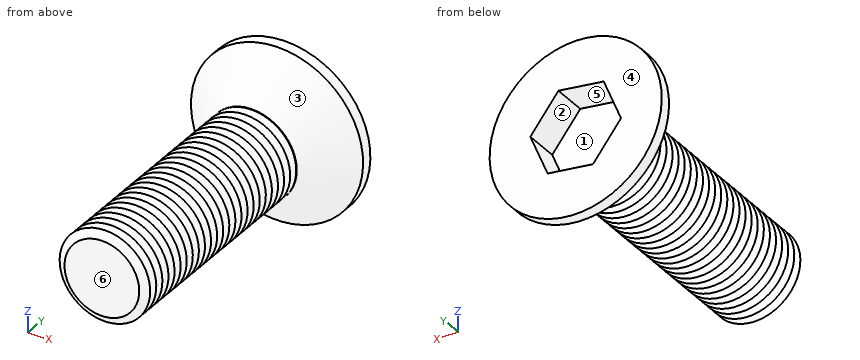
```python
from build123d import *

# Parameters (mm, degrees)
CUT_EXTRUDE_1_DEPTH = 3


with BuildPart() as part:
    # 草图1 → 旋转1 (revolve)
    with BuildSketch(Plane.XY, mode=Mode.PRIVATE) as revolve_1_sk:
        Polygon((7.6, 25), (0, 25), (0, 0), (3.3, 0), (4, 0.416910771), (3.3, 0.833821542), (4, 1.250732313), (3.3, 1.667643084), (4, 2.084553856), (3.3, 2.501464627), (4, 2.918375398), (3.3, 3.335286169), (4, 3.75219694), (3.3, 4.169107711), (4, 4.586018482), (3.3, 5.002929253), (4, 5.419840024), (3.3, 5.836750796), (4, 6.253661567), (3.3, 6.670572338), (4, 7.087483109), (3.3, 7.50439388), (4, 7.921304651), (3.3, 8.338215422), (4, 8.755126193), (3.3, 9.172036964), (4, 9.588947736), (3.3, 10.005858507), (4, 10.422769278), (3.3, 10.839680049), (4, 11.25659082), (3.3, 11.673501591), (4, 12.090412362), (3.3, 12.507323133), (4, 12.924233904), (3.3, 13.341144675), (4, 13.758055447), (3.3, 14.174966218), (4, 14.591876989), (3.3, 15.00878776), (4, 15.425698531), (3.3, 15.842609302), (4, 16.259520073), (3.3, 16.676430844), (4, 17.093341615), (3.3, 17.510252387), (4, 17.927163158), (3.3, 18.344073929), (4, 18.7609847), (3.3, 19.177895471), (4, 19.594806242), (3.3, 20.011717013), (4, 20.428627784), (4, 20.5), (7.6, 24), align=None)
    revolve(revolve_1_sk.sketch.rotate(Axis((0, 20.5, 0), (0, 1, 0)), 270), axis=Axis((0, 20.5, 0), (0, 1, 0)))

    # 草图3 → 切除-拉伸1 (cut)
    with BuildSketch(Plane(origin=(0, 25, 0), x_dir=(1, 0, 0), z_dir=(0, 1, 0))):
        Polygon((4.003980009, -0.549069595), (2.477498223, 3.193013606), (-1.526481787, 3.742083202), (-4.003980009, 0.549069595), (-2.477498223, -3.193013606), (1.526481787, -3.742083202), align=None)
    extrude(amount=-CUT_EXTRUDE_1_DEPTH, mode=Mode.SUBTRACT)


solid = part.part
```
Check sheet for the modelled part. Datum: model origin and axes. Units: mm. Face numbers are marked on the shaded views. A direction names the side the tool comes from. Round coordinates to 2 decimals unless told otherwise and drop trailing zeros. Answer as CSV lines item,"result". Start each with the question number.
1) Tool access check on the marked faces 5 and 6. Record the directions out of +Z, -Z, +X, -X, +Y, -Y that give a thin tool (end or side, any length) a straight path to the whole face; none if there is none.
2) Depth check by flat-ended pin: pin 1 (1 mm diameter, centred on y = 17.5, z = 2.5, fed in from +X); pin 2 (2 mm diameter, centred on y = 20, z = 4, fed in from +X); pin 3 (5 mm diameter, centred on x = -1.5, z = -2.5, fed in from +Y); pin 4 (2 mm diameter, centred on x = -1.5, z = -1, fed in from +Y). Enter the tip coordinate at first touch or a pass-through.
3) Draft check along X on the marked faces 1, 2, 3 and 4. Enter one of: +X half, -X half, draft (parallel to the pull), parting line (faces both ways), or undercut.
4) Scan lines: probe 1 along Y at (x, z) = (-1.25, -1.75); probe 2 along Y at (x, z) = (-5.25, -1); probe 3 along X at (y, z) = (8, -0.25). Record each from-to range of solid material in increasing order.
Determined:
1,face 5,"+Y"
1,face 6,"+Z, -Z, +X, -X, -Y"
2,pin 1,"x = 3.33"
2,pin 2,"x = 2.65"
2,pin 3,"y = 25"
2,pin 4,"y = 22"
3,face 1,"undercut"
3,face 2,"undercut"
3,face 3,"parting line"
3,face 4,"draft"
4,probe 1,"0 to 22"
4,probe 2,"21.81 to 25"
4,probe 3,"-3.86 to 3.86"
